Here's how the part is built. I have some questions about the finished solid (model axes, mm). A direction names the side the tool comes from. Coordinates: 2 decimals unless noted, no trailing zeros. Write each loop counter-clockwise with the first axis right and the second up, starting at its lowest first coordinate (ties: lowest second). Pieces come first, ordered by that corner, then holes. Notation, with made-up numbers: (32, 49) -> (62, 49) arc R25 ccw to (62, 83) -> close; hole circle Ø6 at (-25.5, 38). An arc over 180 degrees is marked (long way). Use a Markdown table: item, result. Add a question column.
Item 1: If I drill on line 1 along X through (y, z) = (-0.25, 3.5); line 2 along Z through (x, y) = (1.25, 1); line 3 along Y through (x, z) = (0.5, 4.25), over which ranges is the centre line in solid material (lowest first)? Write a range as from..to.
Item 2: Imagine slicing it at D-D, the plane x = -2. Write out the boundary of the cut face in (y, z), and give its area (3 significant figures).
Item 3: Imagine slicing it at C-C, the plane z = 26. Write out the boundary of the cut face in (x, y).
Item 4: Imagine slicing it at B-B, the plane x = 1.25. Write out the boundary of the cut face in (y, z), and give its area (3 significant figures).
Item 5: On a 3-axis mill with a long thin cutter (end or side, diameter ignored), from which of +Z, -Z, +X, -X, +Y, -Y can I reach the whole of each face in a straight line? I mean faces 1 (the cylindrical face through (0, 2.1, 2.5)), 2 (the flat face through (0, 0, 30)). Say none if no direction works.
Item 6: If we mould it in two halves opening along X, with no side actions, what happens to faces 3 (the flat face through (-1.6, 0, 2)), 4 (the cylindrical face through (0.1, -3.6, 14.8)), 5 (the flat face through (2, 0, 0))? For each: pulls with the +X half, pulls with the -X half, needs draft (parallel to the pull), parting line crosses it, or undercut.
Item 7: Will these pins go through, and if not, where does the flat tip stop? pin 1 Ø3 at (x, z) = (-2, 18.5) entering from +Y; pin 2 Ø1.6 at (x, y) = (-0.5, 1) entering from -Z.
Item 8: Imagine slicing it at A-A, the plane y = 1. Write out the boundary of the cut face in (x, z).
Autodesk Fusion 360 part; units mm, degrees
sketch "Sketch1" plane through (0, 0, 0) normal (0, 0, 1) x (1, 0, 0)
  line L0 (1.3229, -1.5) -> (-1.3229, -1.5)
  line L1 (-1.5, -1.3229) -> (-1.5, 1.3229)
  line L2 (-1.3229, 1.5) -> (1.3229, 1.5)
  line L3 (1.5, 1.3229) -> (1.5, -1.3229)
  line L4 (1.5, -1.5) -> (-1.5, 1.5) construction
  line L5 (-1.5, -1.5) -> (1.5, 1.5) construction
  arc A0 (-1.5, -1.3229) -> (1.5, -1.3229) centre (0, 0) ccw
  arc A1 (1.5, 1.3229) -> (-1.5, 1.3229) centre (0, 0) ccw
  line L6 (-3, -1.8028) -> (-3, 1.8028)
  arc A2 (3, 1.8028) -> (-3, 1.8028) centre (0, 0) ccw
  line L7 (3, 1.8028) -> (3, -1.8028)
  arc A3 (-3, -1.8028) -> (3, -1.8028) centre (0, 0) ccw
  dimension "d1" = 4
  dimension "d2" = 3
  dimension "d3" = 3
  dimension "d4" = 1.5
extrude "Extrude1" add sketch "Sketch1" along normal blind 30 contours L0 A0 | L0 L1 L2 L3 A0 A1 | L2 A1 | L6 A2 L7 A3 makes body 1
extrude "Extrude2" cut sketch "Sketch1" along normal blind 5 contours L0 A0 | L0 L1 L2 L3 A0 A1 | L2 A1 bodies 1
sketch "Sketch2" plane through (0, 0, 0) normal (0, 0, 1) x (1, 0, 0)
  line L0 (1.3601, -1.6) -> (-1.3601, -1.6)
  line L1 (-1.6, -1.3601) -> (-1.6, 1.3601)
  line L2 (-1.3601, 1.6) -> (1.3601, 1.6)
  line L3 (1.6, 1.3601) -> (1.6, -1.3601)
  line L4 (1.6, -1.6) -> (-1.6, 1.6) construction
  line L5 (-1.6, -1.6) -> (1.6, 1.6) construction
  arc A0 (-1.6, -1.3601) -> (1.6, -1.3601) centre (0, 0) ccw
  arc A1 (1.6, 1.3601) -> (-1.6, 1.3601) centre (0, 0) ccw
  line L6 (-3.1, -1.8303) -> (-3.1, 1.8303)
  arc A2 (3.1, 1.8303) -> (-3.1, 1.8303) centre (0, 0) ccw
  line L7 (3.1, 1.8303) -> (3.1, -1.8303)
  arc A3 (-3.1, -1.8303) -> (3.1, -1.8303) centre (0, 0) ccw
  dimension "d9" = 4.2
  dimension "d10" = 3.2
  dimension "d11" = 3.2
  dimension "d12" = 1.5
extrude "Extrude3" add sketch "Sketch2" along normal blind 30 separate body contours L0 A0 | L0 L1 L2 L3 A0 A1 | L2 A1 | L6 A2 L7 A3 makes body 2
extrude "Extrude4" cut sketch "Sketch2" along normal blind 5 contours L0 A0 | L0 L1 L2 L3 A0 A1 | L2 A1 bodies 2
hidden bodies 1
Ans:
| question | item | result |
|---|---|---|
| 1 | line 1 | x = -3.1..-1.6, 1.6..3.1 |
| 1 | line 2 | z = 5..30 |
| 1 | line 3 | y = -3.57..-2.04, 2.04..3.57 |
| 2 | outline | (-2.99, 0) -> (2.99, 0) -> (2.99, 30) -> (-2.99, 30) -> close |
| 2 | area | 180 mm^2 |
| 3 | outline | (-3.1, -1.83) arc R3.6 ccw to (3.1, -1.83) -> (3.1, 1.83) arc R3.6 ccw to (-3.1, 1.83) -> close |
| 4 | outline | (-3.38, 0) -> (-1.69, 0) -> (-1.69, 5) -> (1.69, 5) -> (1.69, 0) -> (3.38, 0) -> (3.38, 30) -> (-3.38, 30) -> close |
| 4 | area | 186 mm^2 |
| 5 | face 1 | -Z |
| 5 | face 2 | +Z, +X, -X, +Y, -Y |
| 6 | face 3 | undercut |
| 6 | face 4 | parting line crosses it |
| 6 | face 5 | needs draft |
| 7 | pin 1 | stops at y = 3.57 |
| 7 | pin 2 | stops at z = 5 |
| 8 | outline | (-3.1, 0) -> (-1.6, 0) -> (-1.6, 5) -> (1.6, 5) -> (1.6, 0) -> (3.1, 0) -> (3.1, 30) -> (-3.1, 30) -> close |
